```python
from build123d import *

# Parameters (mm, degrees)
BOSS_EXTRUDE1_DEPTH     = 127
SKETCH2_R               = 14.2875
CUT_EXTRUDE1_DEPTH      = 25.4
SKETCH3_R               = 2.032
CUT_EXTRUDE2_DEPTH      = 1
CUT_EXTRUDE2_DEPTH_BACK = 26.4


with BuildPart() as part:
    # Sketch1 → Boss-Extrude1 (new body)
    with BuildSketch(Plane(origin=(0, 0, 0), x_dir=(-1, 0, 0), z_dir=(0, 0, -1))):
        with BuildLine():
            Line((-12.7, 25.146), (-12.7, -25.146))
            ThreePointArc((-12.7, -25.146), (-12.625605122, -25.325605122), (-12.446, -25.4))
            Line((-12.446, -25.4), (12.446, -25.4))
            ThreePointArc((12.446, -25.4), (12.625605122, -25.325605122), (12.7, -25.146))
            Line((12.7, -25.146), (12.7, 25.146))
            ThreePointArc((12.7, 25.146), (12.625605122, 25.325605122), (12.446, 25.4))
            Line((12.446, 25.4), (-12.446, 25.4))
            ThreePointArc((-12.446, 25.4), (-12.625605122, 25.325605122), (-12.7, 25.146))
        make_face()
        with BuildLine():
            Line((-11.1125, -22.225), (-11.1125, 22.225))
            ThreePointArc((-11.1125, 22.225), (-10.647532015, 23.347532015), (-9.525, 23.8125))
            Line((-9.525, 23.8125), (9.525, 23.8125))
            ThreePointArc((9.525, 23.8125), (10.647532015, 23.347532015), (11.1125, 22.225))
            Line((11.1125, 22.225), (11.1125, -22.225))
            ThreePointArc((11.1125, -22.225), (10.647532015, -23.347532015), (9.525, -23.8125))
            Line((9.525, -23.8125), (-9.525, -23.8125))
            ThreePointArc((-9.525, -23.8125), (-10.647532015, -23.347532015), (-11.1125, -22.225))
        make_face(mode=Mode.SUBTRACT)
    extrude(amount=-BOSS_EXTRUDE1_DEPTH)

    # Sketch2 → Cut-Extrude1 (cut)
    with BuildSketch(Plane(origin=(12.7, 0, 0), x_dir=(0, 0, -1), z_dir=(1, 0, 0))):
        with Locations((-101.6, 0)):
            Circle(SKETCH2_R)
    extrude(amount=-CUT_EXTRUDE1_DEPTH, mode=Mode.SUBTRACT)

    # Sketch3 → Cut-Extrude2 (cut, two sides)
    with BuildSketch(Plane(origin=(12.7, 0, 0), x_dir=(0, 0, -1), z_dir=(1, 0, 0))) as cut_extrude2_sk:
        with Locations((-44.45, -19.05)):
            Circle(SKETCH3_R)
        with Locations((-44.45, -6.35)):
            Circle(SKETCH3_R)
        with Locations((-44.45, 19.05)):
            Circle(SKETCH3_R)
        with Locations((-31.75, 19.05)):
            Circle(SKETCH3_R)
        with Locations((-19.05, 19.05)):
            Circle(SKETCH3_R)
        with Locations((-6.35, 19.05)):
            Circle(SKETCH3_R)
        with Locations((-44.45, 6.35)):
            Circle(SKETCH3_R)
        with Locations((-31.75, -19.05)):
            Circle(SKETCH3_R)
        with Locations((-19.05, -19.05)):
            Circle(SKETCH3_R)
        with Locations((-6.35, -19.05)):
            Circle(SKETCH3_R)
    extrude(amount=CUT_EXTRUDE2_DEPTH, mode=Mode.SUBTRACT)
    extrude(cut_extrude2_sk.sketch, amount=-CUT_EXTRUDE2_DEPTH_BACK, mode=Mode.SUBTRACT)


solid = part.part
```
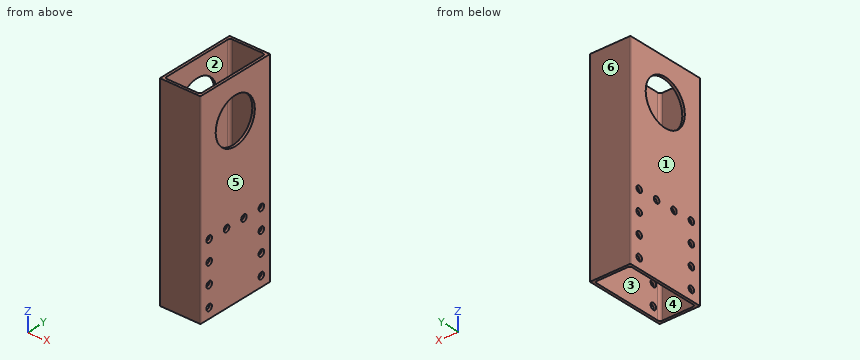
Verification items for the finished model (mm, model axes). Face numbers are marked on the shaded views. A direction names the side the tool comes from. Round coordinates to 2 decimals unless told otherwise and drop trailing zeros. Order: outer loops, then holes, each group sorted by start corner. A loop starts at its lowest first (then second) coordinate and runs counter-clockwise, first axis right, second up. Notation, with made-up numbers: (82.5, 16.25) - (137.5, 16.25) arc R24 ccw to (137.5, 31.25) - close; hole circle Ø11 at (83.5, -9). An arc over 180 degrees is marked (long way). Use CSV: the item, a comma, the result in double quotes. Start each with the question number.
1) Go/stop test with a flat-tipped pin: P1, Ø1.5, axis at x = 9, y = -3.5, coming from the -Z side. Record where the tip stops, or that it passes through.
2) Section check A-A, the plane y = 0. Record the cut outline in (x, z).
3) Thickness scan on L1, parallel to Y at x = -11.95, z = 44.45; L2, parallel to Y at x = -12.3, z = 31.75; L3, parallel to Y at x = 3.5, z = 85.5. Record the ranges inside material, lowest first.
4) Access from +Z, -Z, +X, -X, +Y, -Y to the whole of each face (thin tool, end or side, straight path). Record for the marked faces 1 and 2.
5) Mould release check, pull along Y, two halves, no side actions. Record for the marked faces 3, 4, 5 and 6: +Y half, -Y half, draft (parallel to the pull), parting line (faces both ways), or undercut.
6) Section check C-C, the plane x = 5.5. Record the cut outline in (y, z), plus the area to 3 significant figures.
Answers:
1,P1,"passes through"
2,outline,"(-12.7, 0) - (-11.11, 0) - (-11.11, 87.31) - (-12.7, 87.31) - close; (-12.7, 115.89) - (-11.11, 115.89) - (-11.11, 127) - (-12.7, 127) - close; (11.11, 0) - (12.7, 0) - (12.7, 87.31) - (11.11, 87.31) - close; (11.11, 115.89) - (12.7, 115.89) - (12.7, 127) - (11.11, 127) - close"
3,L1,"y = -25.4 to -21.08, -17.02 to -8.38, -4.32 to 4.32, 8.38 to 17.02, 21.08 to 25.4"
3,L2,"y = -25.4 to -21.08, -17.02 to 17.02, 21.08 to 25.4"
3,L3,"y = -25.4 to -23.81, 23.81 to 25.4"
4,face 1,"+Z, -Z, -X, +Y, -Y"
4,face 2,"+Z, -Z"
5,face 3,"undercut"
5,face 4,"undercut"
5,face 5,"draft"
5,face 6,"+Y half"
6,outline,"(-25.4, 0) - (-23.81, 0) - (-23.81, 127) - (-25.4, 127) - close; (23.81, 0) - (25.4, 0) - (25.4, 127) - (23.81, 127) - close"
6,area,"403 mm²"
